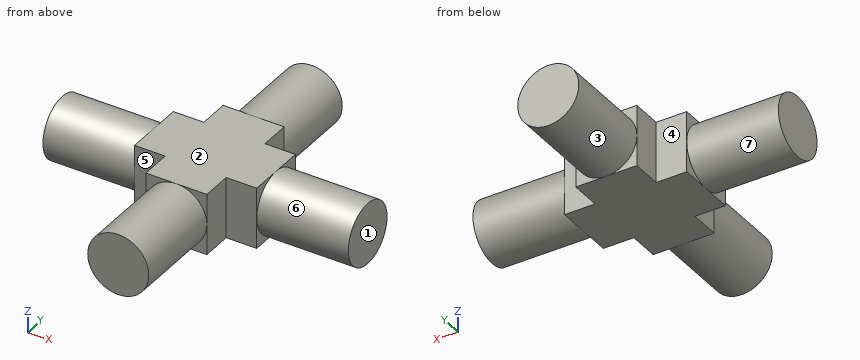
```python
from build123d import *

# Parameters (mm, degrees)
BOSS_EXTRUDE1_DEPTH = 5
SKETCH2_R           = 2.5
BOSS_EXTRUDE2_DEPTH = 7.5
CIRPATTERN1_COUNT   = 4


with BuildPart() as part:
    # Sketch1 → Boss-Extrude1 (new body)
    with BuildSketch(Plane.XY):
        Polygon((-2.5, 2.5), (-5, 2.5), (-5, -2.5), (-2.5, -2.5), (-2.5, -5), (2.5, -5), (2.5, -2.5), (5, -2.5), (5, 2.5), (2.5, 2.5), (2.5, 5), (-2.5, 5), align=None)
    extrude(amount=BOSS_EXTRUDE1_DEPTH)

    # Sketch2 → Boss-Extrude2 (add)
    with BuildSketch(Plane(origin=(0, 5, 0), x_dir=(1, 0, 0), z_dir=(0, 1, 0))):
        with Locations((0, -2.5)):
            Circle(SKETCH2_R)
    boss_extrude2 = extrude(amount=BOSS_EXTRUDE2_DEPTH)

    # CirPattern1: Boss-Extrude2 ×4 about axis
    cirpattern1_axis = Axis((0, 0, 0), (0, 0, 1))
    for i in range(1, CIRPATTERN1_COUNT):
        add(boss_extrude2.rotate(cirpattern1_axis, i * 360 / CIRPATTERN1_COUNT))


solid = part.part
```
For this review, take the finished solid that the model builds, in its own axes (mm). Face numbers are marked on the shaded views. A direction names the side the tool comes from. Round coordinates to 2 decimals unless told otherwise and drop trailing zeros. Write each loop counter-clockwise with the first axis right and the second up, starting at its lowest first coordinate (ties: lowest second). Pieces come first, ordered by that corner, then holes. Notation, with made-up numbers: (72.25, 41.25) -> (105.25, 41.25) arc R23 cw to (105.25, 72.25) -> close; hole circle Ø7 at (37, 27.5). An arc over 180 degrees is marked (long way). One line per question, with ' | ' between items. Start each with the question number.
1) Wall thickness on line 1 along Y through (x, z) = (-4, 2); line 2 along X through (y, z) = (-9.25, 4.25): over which ranges is each line inside the solid? List them lowest first.
2) Mouldability with a two-part tool opening along Z and no side actions: class the marked faces 1, 2 and 3 as +Z half, -Z half, draft (parallel to the pull), parting line (faces both ways), or undercut.
3) Machinability: for the marked faces 4, 5, 6 and 7, which of the approach directions +Z, -Z, +X, -X, +Y, -Y give a long, thin tool a straight path to every point of the face, cutting with its end or side? Answer none if there is none.
4) Add section A-A (y = 1.5). Write out the cut boundary in (x, z), and give its area (3 significant figures).
5) For pin 1 Ø1.5 at (y, z) = (-9, 2) entering from -X; pin 2 Ø0.8 at (x, z) = (4, 1.5) entering from +Y; pin 3 Ø1 at (x, z) = (-9, 3.5) entering from +Y, all flat-tipped, find the tip position at first contact; note any pin that passes through.
6) Add section C-C (x = 6). Write out the cut boundary in (y, z), and give its area (3 significant figures).
7) Add section B-B (z = 4.15). Write out the cut boundary in (x, y).
Reported:
1) line 1: y = -2.5 to 2.5 | line 2: x = -1.79 to 1.79
2) face 1: draft | face 2: +Z half | face 3: parting line
3) face 4: +Z, -Z, -X, +Y | face 5: +Z, -Z, -X, -Y | face 6: +X | face 7: -X
4) outline: (-12.5, 0.5) -> (-5, 0.5) -> (-5, 0) -> (5, 0) -> (5, 0.5) -> (12.5, 0.5) -> (12.5, 4.5) -> (5, 4.5) -> (5, 5) -> (-5, 5) -> (-5, 4.5) -> (-12.5, 4.5) -> close | area: 110 mm²
5) pin 1: stops at x = -2.5 | pin 2: stops at y = 2.5 | pin 3: stops at y = 2.45
6) outline: circle Ø5 at (0, 2.5) | area: 19.6 mm²
7) outline: (-12.5, -1.88) -> (-5, -1.88) -> (-5, -2.5) -> (-2.5, -2.5) -> (-2.5, -5) -> (-1.88, -5) -> (-1.88, -12.5) -> (1.88, -12.5) -> (1.88, -5) -> (2.5, -5) -> (2.5, -2.5) -> (5, -2.5) -> (5, -1.88) -> (12.5, -1.88) -> (12.5, 1.88) -> (5, 1.88) -> (5, 2.5) -> (2.5, 2.5) -> (2.5, 5) -> (1.88, 5) -> (1.88, 12.5) -> (-1.88, 12.5) -> (-1.88, 5) -> (-2.5, 5) -> (-2.5, 2.5) -> (-5, 2.5) -> (-5, 1.88) -> (-12.5, 1.88) -> close
